from build123d import *

# Parameters (mm, degrees)
F0_W     = 12.7
F0_H     = 25.4
F1_DEPTH = 6
F2_W     = 40.6199608326
F2_H     = 25.4
F2_W_2   = 12.7
F3_DEPTH = 3


with BuildPart() as f1:
    # F0 (on Top) → F1 (new body)
    with BuildSketch(Plane.XY):
        with Locations((6.35, 12.7)):
            Rectangle(F0_W, F0_H)
    extrude(amount=F1_DEPTH)



with BuildPart() as f1b:
    # F0 (on Top) → F1, piece 2 (new body)
    with BuildSketch(Plane.XY):
        with Locations((46.99, 12.7)):
            Rectangle(F0_W, F0_H)
    extrude(amount=F1_DEPTH)


with BuildPart() as f1_1:
    add(f1.part)

    add(f1b.part)  # F3 merges F1b
    # F2 (on face) → F3 (join)
    with BuildSketch(Plane.XY.offset(6)):
        with Locations((33.0099804163, 12.7)):
            Rectangle(F2_W, F2_H)
        with Locations((6.35, 12.7)):
            Rectangle(F2_W_2, F2_H)
    extrude(amount=F3_DEPTH)


solid = f1_1.part
The listing builds one solid part. Answer for the finished solid, in the listing's coordinates (mm). A direction names the side the tool comes from. Give positions to 0.01 mm unless a question says otherwise; leave off trailing zeros. Loops run counter-clockwise (first coordinate to the right, second up) from the corner with the lowest first, then second, coordinate; pieces in that order, holes last. Notation, with made-up numbers: (-17, 35.5) - (17, 35.5) arc R16 cw to (17, 54.5) - close; hole circle Ø11 at (6.25, 53.5). An arc over 180 degrees is marked (long way). Answer as a JSON object with one key per item and string values.
1. Find the intervals of material crossed by L1, parallel to X at y = 14.5, z = 5.5; L2, parallel to Z at x = 22, y = 11.75; L3, parallel to X at y = 5, z = 8.5, in increasing order. Write a range as [from, to].
Determined:
{"L1": "[0, 12.7], [40.64, 53.34]", "L2": "[6, 9]", "L3": "[0, 53.32]"}
2. Flat-ended cylindrical pins translate along their axes: pin 1 Ø3 at (y, z) = (10, 2) entering from -X; pin 2 Ø7.5 at (x, y) = (20.5, 13.5) entering from -Z; pin 3 Ø1.5 at (y, z) = (17, 7.5) entering from +X. Find the tip coordinate at first contact, or state that the pin passes through.
Determined:
{"pin 1": "x = 0", "pin 2": "z = 6", "pin 3": "x = 53.32"}
3. A cutting plane is placed at A-A (z = 2.5). Write down the section's boundary in (x, y).
Determined:
{"outline": "(0, 0) - (12.7, 0) - (12.7, 25.4) - (0, 25.4) - close; (40.64, 0) - (53.34, 0) - (53.34, 25.4) - (40.64, 25.4) - close"}
4. For faces 1 (the flat face through (12.7, 13, 3)), 2 (the flat face through (53.34, 13, 3)), determine the directions among +Z, -Z, +X, -X, +Y, -Y from which every point of the face is accessible in a straight line to the end or side of a thin tool.
Determined:
{"face 1": "-Z, +Y, -Y", "face 2": "+Z, -Z, +X, +Y, -Y"}
5. A cutting plane is placed at C-C (x = 35). Write down the section's boundary in (y, z), then the cut area to 3 significant figures.
Determined:
{"outline": "(0, 6) - (25.4, 6) - (25.4, 9) - (0, 9) - close", "area": "76.2 mm²"}
